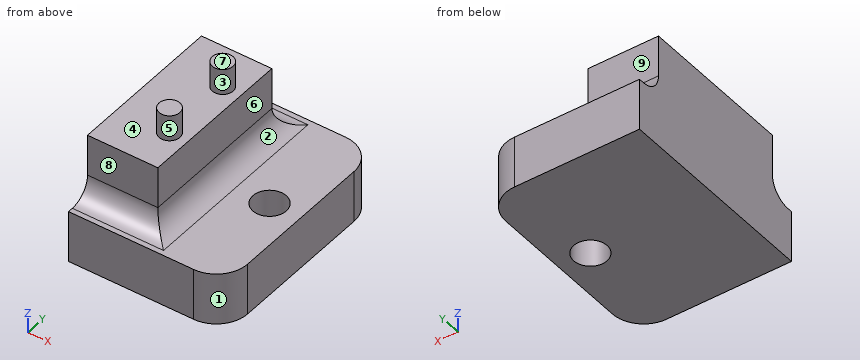
from build123d import *

# Parameters (mm, degrees)
CROQUIS1_R              = 1.6
SALIENTE_EXTRUIR1_DEPTH = 5
CROQUIS2_W              = 6.75
CROQUIS2_H              = 15
SALIENTE_EXTRUIR2_DEPTH = 6
REDONDEO1_R             = 2
CROQUIS3_R              = 1
SALIENTE_EXTRUIR3_DEPTH = 2.5


with BuildPart() as part:
    # Croquis1 → Saliente-Extruir1 (new body)
    with BuildSketch(Plane.XY):
        with BuildLine():
            Line((0, 0), (12, 0))
            ThreePointArc((12, 0), (14.121320344, 0.878679656), (15, 3))
            Line((15, 3), (15, 17))
            ThreePointArc((15, 17), (14.121320344, 19.121320344), (12, 20))
            Line((12, 20), (0, 20))
            Line((0, 20), (0, 0))
        make_face()
        with Locations((12, 10)):
            Circle(CROQUIS1_R, mode=Mode.SUBTRACT)
    extrude(amount=SALIENTE_EXTRUIR1_DEPTH)

    # Croquis2 → Saliente-Extruir2 (add)
    with BuildSketch(Plane.XY.offset(5)):
        with Locations((3.375, 10)):
            Rectangle(CROQUIS2_W, CROQUIS2_H)
    extrude(amount=SALIENTE_EXTRUIR2_DEPTH)

    # Redondeo1
    redondeo1_edges = [part.edges().sort_by_distance(p)[0] for p in [
        (3.375, 2.5, 5),
        (6.75, 10, 5),
        (3.375, 17.5, 5),
    ]]
    fillet(redondeo1_edges, radius=REDONDEO1_R)

    # Croquis3 → Saliente-Extruir3 (add)
    with BuildSketch(Plane.XY.offset(11)):
        with Locations((4.95023571, 13.5)):
            Circle(CROQUIS3_R)
        with Locations((4.95023571, 6.5)):
            Circle(CROQUIS3_R)
    extrude(amount=SALIENTE_EXTRUIR3_DEPTH)


solid = part.part
The model under review builds one solid part; all positions refer to its coordinate system, in mm. Face numbers are marked on the shaded views. A direction names the side the tool comes from. Round coordinates to 2 decimals unless told otherwise and drop trailing zeros. Loops run counter-clockwise (first coordinate to the right, second up) from the corner with the lowest first, then second, coordinate; pieces in that order, holes last. Notation, with made-up numbers: M 64,-20.5 L 87,-20.5 A27 ccw 87,14.5 Z; hole C -2.5,-15 d5. An arc over 180 degrees is marked long. Answer as a JSON object with one key per item and string values.
Item 1: Clearance check with flat-ended pins moving along their axes: P1, Ø5, axis at y = 12, z = 10.5, coming from the +X side; P2, Ø2, axis at x = 4, z = 8, coming from the +Y side; P3, Ø5, axis at x = 12, y = 10, coming from the +Z side. State where each tip first meets the part, or that it passes through.
Check sheet entries:
{"P1": "x = 6.75", "P2": "y = 17.5", "P3": "z = 5"}
Item 2: We need section C-C, the plane y = 13.5. State the section outline as (x, z) points, and give its area (3 significant figures).
Check sheet entries:
{"outline": "M 0,0 L 15,0 L 15,5 L 8.75,5 A2 cw 6.75,7 L 6.75,11 L 5.95,11 L 5.95,13.5 L 3.95,13.5 L 3.95,11 L 0,11 Z", "area": "121 mm2"}
Item 3: We need section B-B, the plane z = 1.75. State the section outline as (x, y) points, and give its area (3 significant figures).
Check sheet entries:
{"outline": "M 0,0 L 12,0 A3 ccw 15,3 L 15,17 A3 ccw 12,20 L 0,20 Z; hole C 12,10 d3.2", "area": "288 mm2"}
Item 4: The part is to be moulded in two halves that separate along Y. For the marked faces 1, 2, 3 and 4, say which applies: +Y half, -Y half, draft (parallel to the pull), parting line (faces both ways), or undercut.
Check sheet entries:
{"face 1": "-Y half", "face 2": "draft", "face 3": "undercut", "face 4": "undercut"}
Item 5: We need section D-D, the plane x = 2.75. State the section outline as (y, z) points.
Check sheet entries:
{"outline": "M 0,0 L 20,0 L 20,5 L 19.5,5 A2 cw 17.5,7 L 17.5,11 L 2.5,11 L 2.5,7 A2 cw 0.5,5 L 0,5 Z"}
Item 6: We need section A-A, the plane y = 10. State the section outline as (x, z) points.
Check sheet entries:
{"outline": "M 0,0 L 10.4,0 L 10.4,5 L 8.75,5 A2 cw 6.75,7 L 6.75,11 L 0,11 Z; M 13.6,0 L 15,0 L 15,5 L 13.6,5 Z"}
Item 7: For line 1 along Y through (x, z) = (12, 2.4); line 2 along Z through (x, y) = (13.5, 7); line 3 along Y through (x, z) = (4.5, 12.5), list the stretches that pass through material, from the lowest coordinate up.
Check sheet entries:
{"line 1": "0 to 8.4, 11.6 to 20", "line 2": "0 to 5", "line 3": "5.61 to 7.39, 12.61 to 14.39"}
Item 8: Tool access review of the marked faces 5, 6, 7, 8 and 9: name each direction out of +Z, -Z, +X, -X, +Y, -Y from which nothing blocks a thin tool from reaching the whole face with its end or side.
Check sheet entries:
{"face 5": "+Z", "face 6": "+Z, +X, +Y, -Y", "face 7": "+Z, +X, -X, +Y, -Y", "face 8": "+Z, +X, -X, -Y", "face 9": "+Z, +X, -X, +Y"}
